Design review of the part shown in the three views and the two pictorial views. Dimensions are in mm from the part's minimum x, y and z. Give positions to 0.01 mm unless a question says otherwise; leave off trailing zeros. Loops run counter-clockwise (first coordinate to the right, second up) from the corner with the lowest first, then second, coordinate; pieces in that order, holes last. Notation, with made-up numbers: (61, 61.5) - (79, 61.5) arc R21 cw to (79, 80.5) - close; hole circle Ø5 at (54.25, 78). An arc over 180 degrees is marked (long way). Answer in a Markdown table with one row per item.
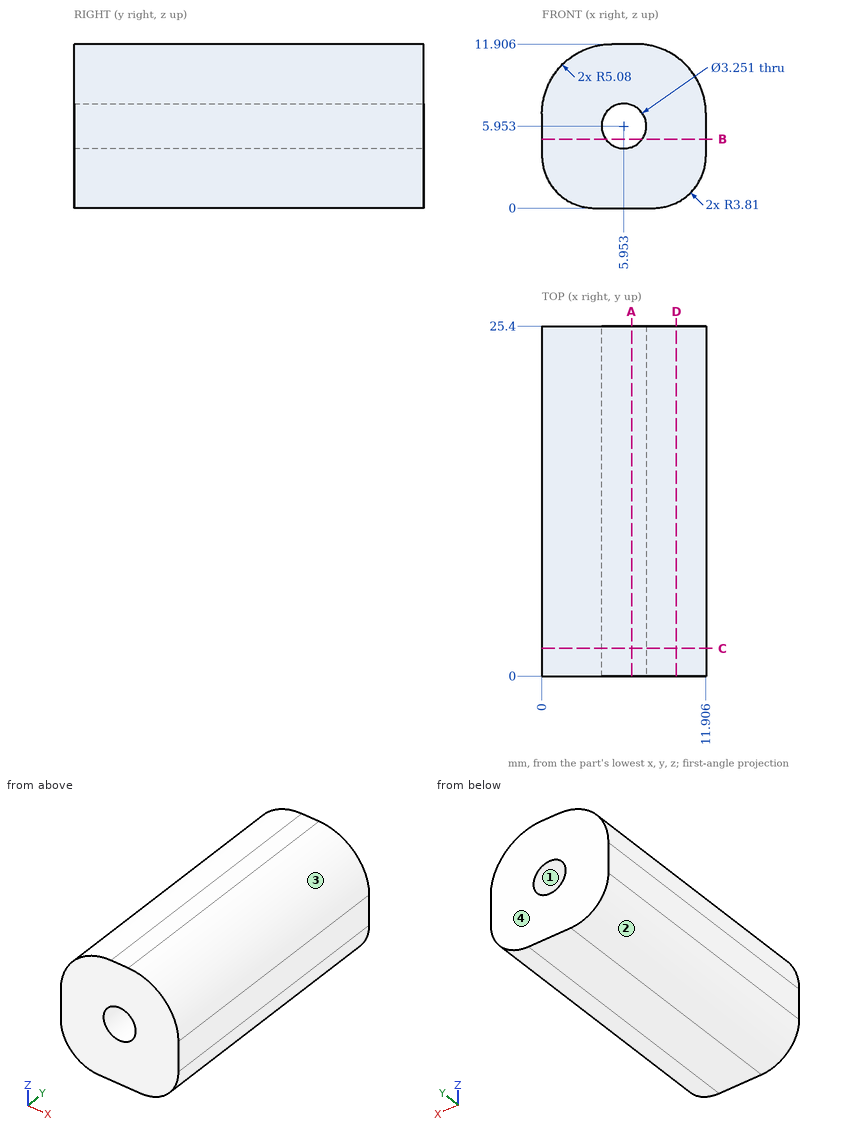
1. Wall thickness on line 1 (Z direction, x = 7, y = 22); line 2 (Z direction, x = 5.5, y = 18.25) (1 decimal); line 3 (Z direction, x = 11.25, y = 8) (1 decimal): over which ranges is each line inside the solid? List them lowest first. Write a range as [from, to].
Values:
| item | result |
|---|---|
| line 1 | z = [0, 4.71], [7.2, 11.9] |
| line 2 | z = [0, 4.4], [7.5, 11.9] |
| line 3 | z = [1.7, 9.3] |
2. We need section A-A, the plane x = 6.5. Give the boundary of the cut face in (y, z), and give its area (3 significant figures).
Values:
| item | result |
|---|---|
| outline | (0, 0) - (25.4, 0) - (25.4, 4.42) - (0, 4.42) - close; (0, 7.48) - (25.4, 7.48) - (25.4, 11.91) - (0, 11.91) - close |
| area | 225 mm^2 |
3. Clearance check with flat-ended pins moving along their axes: pin 1 (1.5 mm diameter, centred on x = 2.5, y = 15.5, fed in from +Z) (1 decimal); pin 2 (2 mm diameter, centred on x = 1.5, y = 22.5, fed in from +Z). State where each tip first meets the part, or that it passes through.
Values:
| item | result |
|---|---|
| pin 1 | stops at z = 11.6 |
| pin 2 | stops at z = 11.2 |
4. We need section C-C, the plane y = 2. Give the boundary of the cut face in (x, z).
Values:
| item | result |
|---|---|
| outline | (0, 3.81) arc R3.81 ccw to (3.81, 0) - (8.1, 0) arc R3.81 ccw to (11.91, 3.81) - (11.91, 6.83) arc R5.08 ccw to (6.83, 11.91) - (5.08, 11.91) arc R5.08 ccw to (0, 6.83) - close; hole circle Ø3.25 at (5.95, 5.95) |
5. We need section D-D, the plane x = 9.75. Give the boundary of the cut face in (y, z), and give its area (3 significant figures).
Values:
| item | result |
|---|---|
| outline | (0, 0.38) - (25.4, 0.38) - (25.4, 10.98) - (0, 10.98) - close |
| area | 269 mm^2 |
6. We need section B-B, the plane z = 5. Give the boundary of the cut face in (x, y).
Values:
| item | result |
|---|---|
| outline | (0, 0) - (4.64, 0) - (4.64, 25.4) - (0, 25.4) - close; (7.27, 0) - (11.91, 0) - (11.91, 25.4) - (7.27, 25.4) - close |
7. Mouldability with a two-part tool opening along X and no side actions: class the marked faces 1, 2, 3 and 4 as released by +X, released by -X, zero draft, split by the parting line, or undercut.
Values:
| item | result |
|---|---|
| face 1 | undercut |
| face 2 | released by -X |
| face 3 | released by +X |
| face 4 | zero draft |
